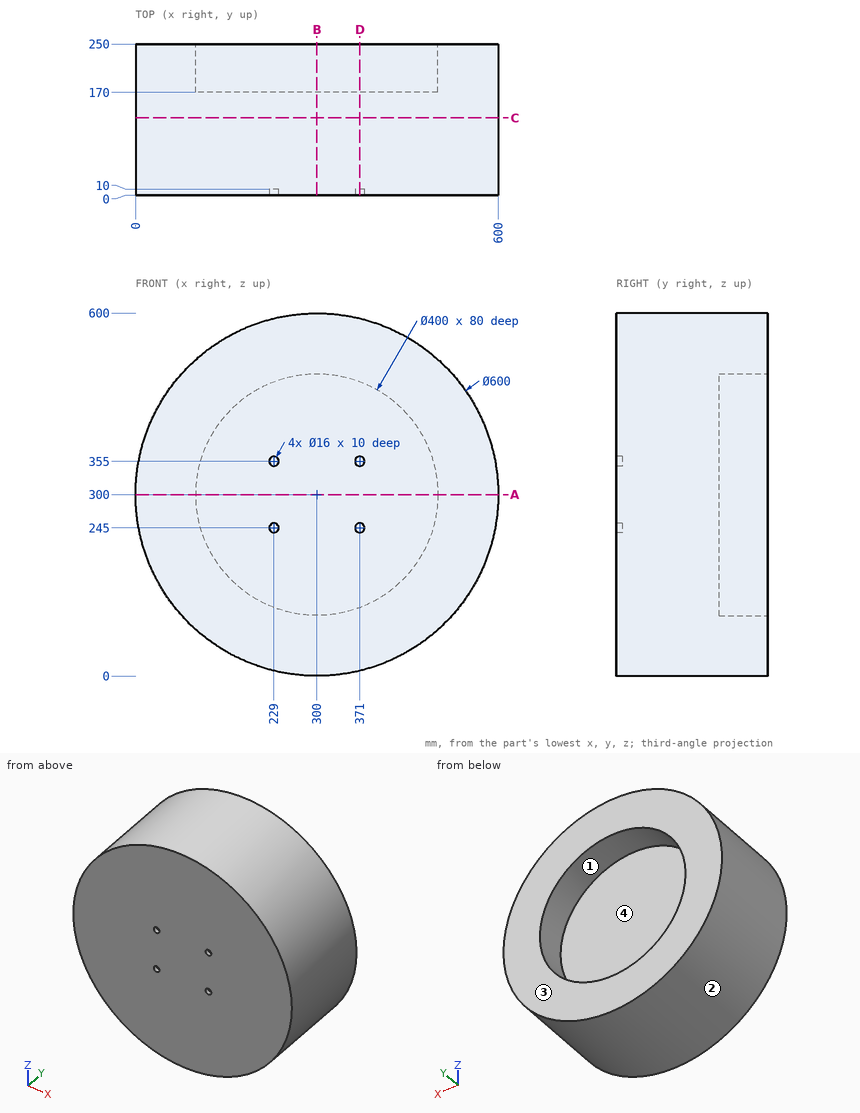
Check sheet for the drawn part. Datum: minimum x, y, z corner. Units: mm. Round coordinates to 2 decimals unless told otherwise and drop trailing zeros. Loops run counter-clockwise (first coordinate to the right, second up) from the corner with the lowest first, then second, coordinate; pieces in that order, holes last. Notation, with made-up numbers: (-26, 35) - (22, 35) arc R29 cw to (22, 71) - close; hole circle Ø3 at (10, -32.5). An arc over 180 degrees is marked (long way). Write item = value, one per line. Start each with the question number.
1. Section check A-A on z = 300. Enter the section's corners in (x, y).
2. Section check D-D on x = 371. Enter the section's corners in (y, z).
3. Thickness scan on line 1 (Z direction, x = 229, y = 5); line 2 (X direction, y = 183.5, z = 300.5). Record the ranges inside material, lowest first.
4. Depth check by flat-ended pin: pin 1 (13 mm diameter, centred on x = 371, z = 355, fed in from +Y); pin 2 (2 mm diameter, centred on x = 502.5, y = 63.5, fed in from -Z); pin 3 (1 mm diameter, centred on x = 95, y = 135.5, fed in from +Z); pin 4 (21 mm diameter, centred on x = 229, z = 355, fed in from -Y). Enter the tip coordinate at first touch or a pass-through.
5. Section check B-B on x = 300. Enter the section's corners in (y, z).
6. Mould release check, pull along X, two halves, no side actions. Record for the marked faces 1, 2, 3 and 4: released by +X, released by -X, zero draft, split by the parting line, or undercut.
7. Section check C-C on y = 128. Enter the section's corners in (x, z), then the cut area to 3 significant figures.
Working result:
q1.outline = (0, 0) - (600, 0) - (600, 250) - (500, 250) - (500, 170) - (100, 170) - (100, 250) - (0, 250) - close
q2.outline = (0, 8.52) - (250, 8.52) - (250, 113.03) - (170, 113.03) - (170, 486.97) - (250, 486.97) - (250, 591.48) - (0, 591.48) - (0, 363) - (10, 363) - (10, 347) - (0, 347) - (0, 253) - (10, 253) - (10, 237) - (0, 237) - close
q3.line_1 = 8.52 to 237, 253 to 347, 363 to 591.48
q3.line_2 = 0 to 100, 500 to 600
q4.pin_1 = 170
q4.pin_2 = 77.74
q4.pin_3 = 519.5
q4.pin_4 = 0
q5.outline = (0, 0) - (250, 0) - (250, 100) - (170, 100) - (170, 500) - (250, 500) - (250, 600) - (0, 600) - close
q6.face_1 = undercut
q6.face_2 = split by the parting line
q6.face_3 = zero draft
q6.face_4 = undercut
q7.outline = circle Ø600 at (300, 300)
q7.area = 283,000 mm^2
